from build123d import *

# Parameters (mm, degrees)
R_VOLUTION1_ANGLE            = 90
ESQUISSE6_R                  = 3.75
BOSS_EXTRU_1_DEPTH           = 10
R_P_TITION_CIRCULAIRE2_COUNT = 2
R_P_TITION_CIRCULAIRE2_ANGLE = 270
R_P_TITION_CIRCULAIRE3_COUNT = 2
R_P_TITION_CIRCULAIRE3_ANGLE = 90


with BuildPart() as part:
    # Esquisse2 → Révolution1 (revolve)
    with BuildSketch(Plane.XY):
        with BuildLine():
            Line((30, 0), (47.131260288, 0))
            add(Edge.make_bspline(
                [(47.131260288, 0), (50.337430192, -76.684539626), (136.959304806, -31.563871951), (150, -100.45024926)],
                knots=[0, 0, 0, 0, 1, 1, 1, 1], degree=3))
            Line((150, -100.45024926), (145, -100.45024926))
            Line((145, -100.45024926), (145, -115.45024926))
            Line((145, -115.45024926), (135, -115.45024926))
            Line((135, -115.45024926), (135, -100.45024926))
            Line((135, -100.45024926), (130, -100.45024926))
            add(Edge.make_bspline(
                [(30, 0), (52.696130576, -79.217712587), (124.807660959, -82.686229226), (130, -100.45024926)],
                knots=[0, 0, 0, 0, 1, 1, 1, 1], degree=3))
        make_face()
    revolve(axis=Axis((0, 55, 0), (0, -1, 0)), revolution_arc=R_VOLUTION1_ANGLE)

    # Esquisse6 → Boss.-Extru.1 (add)
    with BuildSketch(Plane.ZY):
        with Locations(Location((40, -8.5, 0), (0, 0, 180))):
            Circle(ESQUISSE6_R)
        with Locations(Location((71.95431642, -52.883306602, 0), (0, 0, 180))):
            Circle(ESQUISSE6_R)
        with Locations(Location((125, -80, 0), (0, 0, 180))):
            Circle(ESQUISSE6_R)
    extrude(amount=BOSS_EXTRU_1_DEPTH)


with BuildPart() as r_p_tition_circulaire2_1:
    # Répétition circulaire2: pattern copy
    add(part.part.rotate(Axis((0, 55, 0), (0, -1, 0)), 1 * R_P_TITION_CIRCULAIRE2_ANGLE / (R_P_TITION_CIRCULAIRE2_COUNT - 1)))


with BuildPart() as part_1:
    add(part.part)

    # Combiner3: cut Répétition circulaire2_1
    add(r_p_tition_circulaire2_1.part, mode=Mode.SUBTRACT)


with BuildPart() as r_p_tition_circulaire3_1:
    # Répétition circulaire3: pattern copy
    add(part_1.part.rotate(Axis((0, 55, 0), (0, -1, 0)), 1 * R_P_TITION_CIRCULAIRE3_ANGLE / (R_P_TITION_CIRCULAIRE3_COUNT - 1)))


with BuildPart() as part_2:
    add(part_1.part)

    # Combiner4: union Répétition circulaire3_1
    add(r_p_tition_circulaire3_1.part)

    # Lissage2: read off the stored shape, not the designer's step
    # Lissage2: loft between two sections, ruled curve by curve
    lissage2_from = [
        Edge.make_bspline([(-10.141415638, -19.056019087, 58), (-8.212976489, -19.056019087, 58), (-4.745525631, -19.056019087, 58), (0.097340365, -19.056019087, 58), (4.940206361, -19.056019087, 58), (8.407657219, -19.056019087, 58), (10.992070669, -19.056019087, 58), (12.368530298, -19.277794454, 58), (14.347229759, -20.43033769, 58), (15.825485799, -22.4031348, 58), (16.381152507, -24.915194071, 58), (15.825485799, -27.427253342, 58), (14.347229759, -29.400050453, 58), (12.368530298, -30.552593688, 58), (10.992070669, -30.774369055, 58), (8.407657219, -30.774369055, 58), (4.940206361, -30.774369055, 58), (0.097340365, -30.774369055, 58), (-4.745525631, -30.774369055, 58), (-8.212976489, -30.774369055, 58), (-10.797389939, -30.774369055, 58), (-12.173849568, -30.552593688, 58), (-14.152549029, -29.400050453, 58), (-15.630805069, -27.427253342, 58), (-16.186471777, -24.915194071, 58), (-15.630805069, -22.4031348, 58), (-14.152549029, -20.43033769, 58), (-12.173849568, -19.277794454, 58), (-10.797389939, -19.056019087, 58), (-10.141415638, -19.056019087, 58)], [0, 0, 0, 0, 0.074390756, 0.148781511, 0.223172267, 0.297563023, 0.297563023, 0.322867645, 0.348172267, 0.373476889, 0.398781511, 0.424086134, 0.449390756, 0.474695378, 0.5, 0.5, 0.574390756, 0.648781511, 0.723172267, 0.797563023, 0.797563023, 0.822867645, 0.848172267, 0.873476889, 0.898781511, 0.924086134, 0.949390756, 0.974695378, 1, 1, 1, 1], 3),
    ]
    lissage2_to = [
        Edge.make_bspline([(-13.646593818, -29.959479994, 47), (-11.606942776, -29.959479994, 47), (-7.235758652, -29.959479994, 47), (0, -29.959479994, 47), (7.235758652, -29.959479994, 47), (11.606942776, -29.959479994, 47), (14.340397752, -29.959479994, 47), (15.598489603, -30.279278409, 47), (16.997996562, -31.3442136, 47), (17.857241012, -32.768726587, 47), (18.146490081, -34.362953291, 47), (17.857241012, -35.957179995, 47), (16.997996562, -37.381692982, 47), (15.598489603, -38.446628173, 47), (14.340397752, -38.766426588, 47), (11.606942776, -38.766426588, 47), (7.235758652, -38.766426588, 47), (0, -38.766426588, 47), (-7.235758652, -38.766426588, 47), (-11.606942776, -38.766426588, 47), (-14.340397752, -38.766426588, 47), (-15.598489603, -38.446628173, 47), (-16.997996562, -37.381692982, 47), (-17.857241012, -35.957179995, 47), (-18.146490081, -34.362953291, 47), (-17.857241012, -32.768726587, 47), (-16.997996562, -31.3442136, 47), (-15.598489603, -30.279278409, 47), (-14.340397752, -29.959479994, 47), (-13.646593818, -29.959479994, 47)], [0, 0, 0, 0, 0.074390756, 0.148781511, 0.223172267, 0.297563023, 0.297563023, 0.322867645, 0.348172267, 0.373476889, 0.398781511, 0.424086134, 0.449390756, 0.474695378, 0.5, 0.5, 0.574390756, 0.648781511, 0.723172267, 0.797563023, 0.797563023, 0.822867645, 0.848172267, 0.873476889, 0.898781511, 0.924086134, 0.949390756, 0.974695378, 1, 1, 1, 1], 3),
    ]
    lissage2 = Solid(Shell([*[Face.make_surface_from_curves(lissage2_from[k], lissage2_to[k]) for k in range(1)], Face(Wire(lissage2_from)), Face(Wire(lissage2_to))]))
    add(lissage2)

    # Lissage2 2: loft between two sections, ruled curve by curve
    lissage2_2_from = [
        Edge.make_bspline([(-10.141415638, -19.056019087, 58), (-8.212976489, -19.056019087, 58), (-4.745525631, -19.056019087, 58), (0.097340365, -19.056019087, 58), (4.940206361, -19.056019087, 58), (8.407657219, -19.056019087, 58), (10.992070669, -19.056019087, 58), (12.368530298, -19.277794454, 58), (14.347229759, -20.43033769, 58), (15.825485799, -22.4031348, 58), (16.381152507, -24.915194071, 58), (15.825485799, -27.427253342, 58), (14.347229759, -29.400050453, 58), (12.368530298, -30.552593688, 58), (10.992070669, -30.774369055, 58), (8.407657219, -30.774369055, 58), (4.940206361, -30.774369055, 58), (0.097340365, -30.774369055, 58), (-4.745525631, -30.774369055, 58), (-8.212976489, -30.774369055, 58), (-10.797389939, -30.774369055, 58), (-12.173849568, -30.552593688, 58), (-14.152549029, -29.400050453, 58), (-15.630805069, -27.427253342, 58), (-16.186471777, -24.915194071, 58), (-15.630805069, -22.4031348, 58), (-14.152549029, -20.43033769, 58), (-12.173849568, -19.277794454, 58), (-10.797389939, -19.056019087, 58), (-10.141415638, -19.056019087, 58)], [0, 0, 0, 0, 0.074390756, 0.148781511, 0.223172267, 0.297563023, 0.297563023, 0.322867645, 0.348172267, 0.373476889, 0.398781511, 0.424086134, 0.449390756, 0.474695378, 0.5, 0.5, 0.574390756, 0.648781511, 0.723172267, 0.797563023, 0.797563023, 0.822867645, 0.848172267, 0.873476889, 0.898781511, 0.924086134, 0.949390756, 0.974695378, 1, 1, 1, 1], 3),
    ]
    lissage2_2_to = [
        Edge.make_bspline([(-13.646593818, -29.959479994, 47), (-11.606942776, -29.959479994, 47), (-7.235758652, -29.959479994, 47), (0, -29.959479994, 47), (7.235758652, -29.959479994, 47), (11.606942776, -29.959479994, 47), (14.340397752, -29.959479994, 47), (15.598489603, -30.279278409, 47), (16.997996562, -31.3442136, 47), (17.857241012, -32.768726587, 47), (18.146490081, -34.362953291, 47), (17.857241012, -35.957179995, 47), (16.997996562, -37.381692982, 47), (15.598489603, -38.446628173, 47), (14.340397752, -38.766426588, 47), (11.606942776, -38.766426588, 47), (7.235758652, -38.766426588, 47), (0, -38.766426588, 47), (-7.235758652, -38.766426588, 47), (-11.606942776, -38.766426588, 47), (-14.340397752, -38.766426588, 47), (-15.598489603, -38.446628173, 47), (-16.997996562, -37.381692982, 47), (-17.857241012, -35.957179995, 47), (-18.146490081, -34.362953291, 47), (-17.857241012, -32.768726587, 47), (-16.997996562, -31.3442136, 47), (-15.598489603, -30.279278409, 47), (-14.340397752, -29.959479994, 47), (-13.646593818, -29.959479994, 47)], [0, 0, 0, 0, 0.074390756, 0.148781511, 0.223172267, 0.297563023, 0.297563023, 0.322867645, 0.348172267, 0.373476889, 0.398781511, 0.424086134, 0.449390756, 0.474695378, 0.5, 0.5, 0.574390756, 0.648781511, 0.723172267, 0.797563023, 0.797563023, 0.822867645, 0.848172267, 0.873476889, 0.898781511, 0.924086134, 0.949390756, 0.974695378, 1, 1, 1, 1], 3),
    ]
    lissage2_2 = Solid(Shell([*[Face.make_surface_from_curves(lissage2_2_from[k], lissage2_2_to[k]) for k in range(1)], Face(Wire(lissage2_2_from)), Face(Wire(lissage2_2_to))]))
    add(lissage2_2)


solid = part_2.part
Design review of the part built by this model. Coordinates are the model's own, in mm. A direction names the side the tool comes from. Give positions to 0.01 mm unless a question says otherwise; leave off trailing zeros. Return JSON: item names as keys, results as strings. Group by question number.
Item 1: The part is to be moulded in two halves that separate along Y. For faces 1 (the cylindrical face through (37.98, -11.66, 4.93)), 2 (the flat face through (-12, -100.45, 147)), 3 (the cylindrical face through (122.98, -83.16, 4.93)), 4 (the flat face through (-72, -53, -10)), say which applies: pulls with the +Y half, pulls with the -Y half, needs draft (parallel to the pull), parting line crosses it, or undercut.
Item 2: Tool access review of faces 5 (the flat face through (40, -9, 10)), 6 (the flat face through (-1, -115.45, 137)), 7 (the cylindrical face through (3.188, -108.055, 144.965)), 8 (the flat face through (0, -25, 58)), 9 (the flat face through (95, -66, 0)): name each direction out of +Z, -Z, +X, -X, +Y, -Y from which nothing blocks a thin tool from reaching the whole face with its end or side.
Item 3: Clearance check with flat-ended pins moving along their axes: pin 1 Ø12 at (x, y) = (71.95, -52.88) entering from -Z; pin 2 Ø3.5 at (x, y) = (-1.5, -26.5) entering from +Z; pin 3 Ø1.5 at (x, y) = (-48.5, -70.5) entering from -Z. State where each tip first meets the part, or that it passes through.
Item 4: Wall thickness on line 1 along X through (y, z) = (-8.5, 4); line 2 along Y through (x, z) = (40, 3.75); line 3 along X through (y, z) = (-80, 7): over which ranges is each line inside the solid? List them lowest first.
Return value:
{
 "1": {"face 1": "undercut", "face 2": "pulls with the -Y half", "face 3": "undercut", "face 4": "needs draft"},
 "2": {"face 5": "-Z", "face 6": "+Z, -Z, +X, -X, -Y", "face 7": "+Z, -Y", "face 8": "+Z, +X, -X, +Y", "face 9": "-Z, +X, +Y, -Y"},
 "3": {"pin 1": "stops at z = 0", "pin 2": "stops at z = 58", "pin 3": "stops at z = 64.75"},
 "4": {"line 1": "x = -47.72 to -32.48, 32.48 to 36.25, 43.75 to 47.72", "line 2": "y = -25.54 to -12.25, -4.75 to 0", "line 3": "x = -142.12 to -98.4, 98.4 to 121.25, 128.75 to 142.12"}
}
